Could you check a few things on this model? Use its own coordinates, in mm. Face numbers are marked on the shaded views. A direction names the side the tool comes from. Give positions to 0.01 mm unless a question says otherwise; leave off trailing zeros. Loops run counter-clockwise (first coordinate to the right, second up) from the corner with the lowest first, then second, coordinate; pieces in that order, holes last. Notation, with made-up numbers: (-38, 18) - (-15, 18) arc R32 cw to (-15, 50) - close; hole circle Ø4 at (6, -10). An arc over 180 degrees is marked (long way). Write each question's results on one line, items separated by ' | '. Start each with the question number.
1) I want a section at B-B, the plane y = -14. Write out the boundary of the cut face in (x, z), and give its area (3 significant figures).
2) I'm going to push flat-ended pins straight in: pin 1 (3 mm diameter, centred on y = -4, z = 3, fed in from -X); pin 2 (1 mm diameter, centred on x = -6.5, z = 2, fed in from +Y); pin 3 (2 mm diameter, centred on x = 7, z = 2.5, fed in from -Y); pin 4 (3 mm diameter, centred on x = 3, y = -12.5, fed in from +Z). Where does each tip first touch, or does it pass through?
3) I want a section at A-A, the plane x = 12.5. Write out the boundary of the cut face in (y, z).
4) If I drill on probe 1 along Y at (x, z) = (11, 1); probe 2 along X at (y, z) = (-12, 1.75); probe 3 along X at (y, z) = (7, 4), over which ranges is the centre line in solid material (lowest first)? Write a range as [from, to].
5) If we mould it in two halves opening along X, with no side actions, what happens to the marked faces 1, 2, 3 and 4? For each: +X half, -X half, draft (parallel to the pull), parting line (faces both ways), or undercut.
6) I want a section at D-D, the plane x = -5. Write out the boundary of the cut face in (y, z).
7) I want a section at C-C, the plane z = 4. Write out the boundary of the cut face in (x, y).
8) On a 3-axis mill with a long thin cutter (end or side, diameter ignored), from which of +Z, -Z, +X, -X, +Y, -Y can I reach the whole of each face in a straight line? I mean the marked faces 5, 6 and 7. Say none if no direction works.
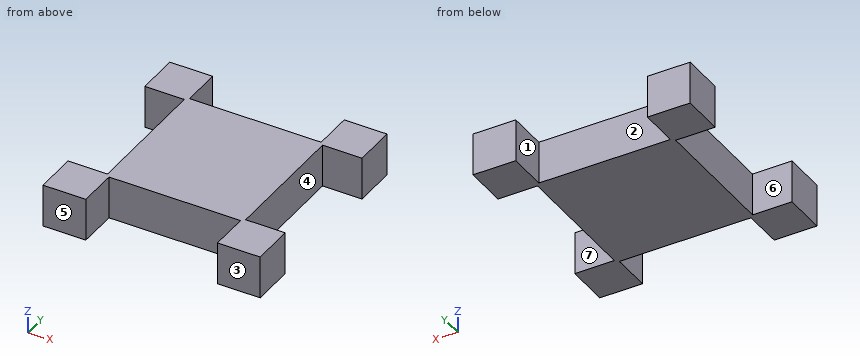
from build123d import *

# Parameters (mm, degrees)
F1_DEPTH = 6.5


with BuildPart() as f1:
    # F0 (on Top) → F1 (new body)
    with BuildSketch(Plane.XY):
        Polygon((-10, 16.5), (-16.5, 16.5), (-16.5, 10), (-10.5, 10), (-10.5, -10), (-16.5, -10), (-16.5, -16.5), (-10, -16.5), (-9.971203, -10.500069), (10.028797, -10.500069), (10, -16.5), (16.5, -16.5), (16.5, -10), (10.5, -10), (10.5, 10), (16.5, 10), (16.5, 16.5), (10, 16.5), (10, 10.5), (-10, 10.5), align=None)
    extrude(amount=F1_DEPTH)


solid = f1.part
Answers:
1) outline: (-16.5, 0) - (-9.99, 0) - (-9.99, 6.5) - (-16.5, 6.5) - close; (10.01, 0) - (16.5, 0) - (16.5, 6.5) - (10.01, 6.5) - close | area: 84.5 mm2
2) pin 1: stops at x = -10.5 | pin 2: stops at y = 10.5 | pin 3: stops at y = -10.5 | pin 4: passes through
3) outline: (-16.5, 0) - (-10, 0) - (-10, 6.5) - (-16.5, 6.5) - close; (10, 0) - (16.5, 0) - (16.5, 6.5) - (10, 6.5) - close
4) probe 1: y = [-16.5, -10], [10, 16.5] | probe 2: x = [-16.5, -9.98], [10.02, 16.5] | probe 3: x = [-10.5, 10.5]
5) face 1: undercut | face 2: undercut | face 3: draft | face 4: +X half
6) outline: (-10.5, 0) - (10.5, 0) - (10.5, 6.5) - (-10.5, 6.5) - close
7) outline: (-16.5, -16.5) - (-10, -16.5) - (-9.97, -10.5) - (10.03, -10.5) - (10, -16.5) - (16.5, -16.5) - (16.5, -10) - (10.5, -10) - (10.5, 10) - (16.5, 10) - (16.5, 16.5) - (10, 16.5) - (10, 10.5) - (-10, 10.5) - (-10, 16.5) - (-16.5, 16.5) - (-16.5, 10) - (-10.5, 10) - (-10.5, -10) - (-16.5, -10) - close
8) face 5: +Z, -Z, +X, -X, -Y | face 6: +Z, -Z, -X | face 7: +Z, -Z, +X
